from build123d import *

# Parameters (mm, degrees)
F0_R     = 72.8
F0_R_2   = 6.85
F0_R_3   = 4
F0_R_4   = 35.95
F1_DEPTH = 10
F2_DEPTH = 4


with BuildPart() as f1:
    # F0 (on Top) → F1 (new body)
    with BuildSketch(Plane.XY):
        Circle(F0_R)
        with Locations((-38.183766, -38.183766)):
            Circle(F0_R_2, mode=Mode.SUBTRACT)
        with Locations((-19.440318, -46.93308)):
            Circle(F0_R_3, mode=Mode.SUBTRACT)
        with Locations((-46.881264, -19.621801)):
            Circle(F0_R_3, mode=Mode.SUBTRACT)
        Circle(F0_R_4, mode=Mode.SUBTRACT)
        with Locations((19.492135, -47.114563)):
            Circle(F0_R_3, mode=Mode.SUBTRACT)
        with Locations((38.183766, -38.183766)):
            Circle(F0_R_2, mode=Mode.SUBTRACT)
        with Locations((46.93308, -19.440318)):
            Circle(F0_R_3, mode=Mode.SUBTRACT)
        with Locations((-46.93308, 19.440318)):
            Circle(F0_R_3, mode=Mode.SUBTRACT)
        with Locations((-38.183766, 38.183766)):
            Circle(F0_R_2, mode=Mode.SUBTRACT)
        with Locations((-19.388502, 46.751597)):
            Circle(F0_R_3, mode=Mode.SUBTRACT)
        with Locations((46.984896, 19.258835)):
            Circle(F0_R_3, mode=Mode.SUBTRACT)
        with Locations((19.440318, 46.93308)):
            Circle(F0_R_3, mode=Mode.SUBTRACT)
        with Locations((38.183766, 38.183766)):
            Circle(F0_R_2, mode=Mode.SUBTRACT)
        Circle(F0_R_4)
    extrude(amount=-F1_DEPTH)

    # F0 (on Top) → F2 (join)
    with BuildSketch(Plane.XY):
        Circle(F0_R_4)
    extrude(amount=F2_DEPTH)


solid = f1.part
Here's how the part is built. I have some questions about the finished solid (model axes, mm). A direction names the side the tool comes from. Give positions to 0.01 mm unless a question says otherwise; leave off trailing zeros. Write each loop counter-clockwise with the first axis right and the second up, starting at its lowest first coordinate (ties: lowest second). Pieces come first, ordered by that corner, then holes. Notation, with made-up numbers: (2, -4) -> (50, -4) arc R9 ccw to (50, 11) -> close; hole circle Ø1 at (54.5, 37.5). An arc over 180 degrees is marked (long way). Use one line per item in the form item = value. Start each with the question number.
1. Thinking about a two-plate mould opening in Y: for faces 1 (the face through (-1, 1, -10)), 2 (the face through (22, -44, -5)), 3 (the face through (-15.78, -71.07, -4.93)), which applies, +Y half, -Y half, draft (parallel to the pull), parting line (faces both ways), or undercut?
2. Will these pins go through, and if not, where does the flat tip stop? pin 1 Ø6 at (y, z) = (56, -8) entering from +X; pin 2 Ø1.5 at (x, z) = (49, -4.5) entering from +Y; pin 3 Ø6 at (x, z) = (37.5, -2.5) entering from +Y.
3. Imagine slicing it at A-A on y = 0. List the corners of the cut face in (x, z) for me, plus the area to 3 significant figures.
4. Imagine slicing it at C-C on y = -40. List the corners of the cut face in (x, z) for me.
5. On a 3-axis mill with a long thin cutter (end or side, diameter ignored), from which of +Z, -Z, +X, -X, +Y, -Y can I reach the whole of each face in a straight line? I mean faces 4 (the face through (32.748, -42.352, -4.93)), 5 (the face through (-33, -15, 0)). Say none if no direction works.
6. Imagine slicing it at B-B on x = -38. List the corners of the cut face in (y, z) for me.
7. If I drill on L1, parallel to X at y = 33, z = -4.5; L2, parallel to X at y = 34, z = -4.5; L3, parallel to Z at x = 45, y = -52, over which ranges is the centre line in solid material (lowest first)?
Entries:
q1.face_1 = draft
q1.face_2 = undercut
q1.face_3 = parting line
q2.pin_1 = 49.91
q2.pin_2 = 54.51
q2.pin_3 = 64.11
q3.outline = (-72.8, -10) -> (72.8, -10) -> (72.8, 0) -> (35.95, 0) -> (35.95, 4) -> (-35.95, 4) -> (-35.95, 0) -> (-72.8, 0) -> close
q3.area = 1,740 mm²
q4.outline = (-60.83, -10) -> (-44.79, -10) -> (-44.79, 0) -> (-60.83, 0) -> close; (-31.58, -10) -> (31.58, -10) -> (31.58, 0) -> (-31.58, 0) -> close; (44.79, -10) -> (60.83, -10) -> (60.83, 0) -> (44.79, 0) -> close
q5.face_4 = +Z, -Z
q5.face_5 = +Z
q6.outline = (-62.1, -10) -> (-45.03, -10) -> (-45.03, 0) -> (-62.1, 0) -> close; (-31.34, -10) -> (31.34, -10) -> (31.34, 0) -> (-31.34, 0) -> close; (45.03, -10) -> (62.1, -10) -> (62.1, 0) -> (45.03, 0) -> close
q7.L1 = -64.89 to -42.66, -33.71 to 33.71, 42.66 to 64.89
q7.L2 = -64.37 to -43.61, -32.76 to 32.76, 43.61 to 64.37
q7.L3 = -10 to 0
